```python
from build123d import *

# Parameters (mm, degrees)
SKETCH_1_R          = 30.5
EXTRUDE_1_DEPTH     = 12.6
SKETCH_2_R          = 32.75
EXTRUDE_2_DEPTH     = 22
SKETCH_3_R          = 29
EXTRUDE_3_DEPTH     = 5
EXTRUDE_START       = -1.1
EXTRUDE_4_DEPTH     = 10.6
SKETCH_5_R          = 1.5
CUT_EXTRUDE_1_DEPTH = 5
SKETCH_6_R          = 27.75
CUT_EXTRUDE_2_DEPTH = 2
CUT_EXTRUDE_START   = -1.2
CUT_EXTRUDE_3_DEPTH = 10.8


with BuildPart() as part:
    # 草图1 → 凸台-拉伸1 (new body)
    with BuildSketch(Plane.XY):
        Circle(SKETCH_1_R)
    extrude(amount=EXTRUDE_1_DEPTH)

    # 草图2 → 凸台-拉伸2 (add)
    with BuildSketch(Plane.XY.offset(12.6)):
        Circle(SKETCH_2_R)
    extrude(amount=EXTRUDE_2_DEPTH)

    # 草图3 → 凸台-拉伸3 (add)
    with BuildSketch(Plane.XY.offset(34.6)):
        Circle(SKETCH_3_R)
    extrude(amount=EXTRUDE_3_DEPTH)

    # 草图4 → 凸台-拉伸4 (add)
    with BuildSketch(Plane(origin=(0, 0, 0), x_dir=(-1, 0, 0), z_dir=(0, 0, -1)).offset(EXTRUDE_START)):
        with BuildLine():
            ThreePointArc((21.25, -21.878928219), (0, -30.5), (-21.25, -21.878928219))
            Line((-21.25, -21.878928219), (-21.25, -36.2))
            Line((-21.25, -36.2), (21.25, -36.2))
            Line((21.25, -36.2), (21.25, -21.878928219))
        make_face()
    extrude(amount=-EXTRUDE_4_DEPTH)

    # 草图5 → 切除-拉伸1 (cut)
    with BuildSketch(Plane.XZ.offset(36.2)):
        with Locations(Location((-18, 6.4, 0), (0, 0, 270))):
            Circle(SKETCH_5_R)
        with Locations(Location((18, 6.4, 0), (0, 0, 90))):
            Circle(SKETCH_5_R)
    extrude(amount=-CUT_EXTRUDE_1_DEPTH, mode=Mode.SUBTRACT)

    # 草图6 → 切除-拉伸2 (cut)
    with BuildSketch(Plane(origin=(0, 0, 0), x_dir=(-1, 0, 0), z_dir=(0, 0, -1))):
        Circle(SKETCH_6_R)
    extrude(amount=-CUT_EXTRUDE_2_DEPTH, mode=Mode.SUBTRACT)

    # 草图7 → 切除-拉伸3 (cut)
    with BuildSketch(Plane(origin=(0, 0, 0), x_dir=(-1, 0, 0), z_dir=(0, 0, -1)).offset(CUT_EXTRUDE_START)):
        with BuildLine():
            ThreePointArc((28.52384967, 10.8), (0, 30.5), (-28.52384967, 10.8))
            Line((-28.52384967, 10.8), (-27.988569095, 10.8))
            ThreePointArc((-27.988569095, 10.8), (0, 30), (27.988569095, 10.8))
            Line((27.988569095, 10.8), (28.52384967, 10.8))
        make_face()
    extrude(amount=-CUT_EXTRUDE_3_DEPTH, mode=Mode.SUBTRACT)


solid = part.part
```
The model under review builds one solid part; all positions refer to its coordinate system, in mm. A direction names the side the tool comes from. Give positions to 0.01 mm unless a question says otherwise; leave off trailing zeros. Write each loop counter-clockwise with the first axis right and the second up, starting at its lowest first coordinate (ties: lowest second). Pieces come first, ordered by that corner, then holes.
(1) Consider section D-D, the plane x = -18. Give the boundary of the cut face in (y, z), and give its area (3 significant figures).
(2) Tool access review of faces 1 (the cylindrical face through (-16.735, -33.735, 5.594)), 2 (the cylindrical face through (31.238, 9.837, 23.446)), 3 (the flat face through (21.25, -29, 6)), 4 (the cylindrical face through (0.505, 29.996, 6.524)), 5 (the flat face through (-21.25, -29, 6)): name each direction out of +Z, -Z, +X, -X, +Y, -Y from which nothing blocks a thin tool from reaching the whole face with its end or side.
(3) Consider section A-A, the plane y = 0. Give the boundary of the cut face in (x, z).
(4) For P1, Ø3, axis at x = 21, y = -22.5, coming from the +Z side; P2, Ø3, axis at y = -9.5, z = 15.5, coming from the +X side; P3, Ø1.5, axis at x = 18, z = 6.5, coming from the -Y side; P4, Ø3, axis at x = 24.5, y = 25, coming from the +Z side, all flat-tipped, find the tip position at first contact; note any pin that passes through.
(5) The part is to be moulded in two halves that separate along X. For faces 6 (the cylindrical face through (13.38, -25.73, 37.06)), 7 (the flat face through (0, 0, 2)), 8 (the flat face through (0.1, 30.2, 12)), say which applies: released by +X, released by -X, zero draft, split by the parting line, or undercut.
(6) To check wall thickness, follow L1, parallel to X at y = -32.6, z = 6.4; L2, parallel to Y at x = 0, z = 0.8; L3, parallel to Y at x = 0, z = 1.3. State the ranges of each line that lie inside material, in increasing order.
(7) Consider section B-B, the plane z = 6.4. Give the boundary of the cut face in (x, y).
(8) Consider section C-C, the plane x = -2. Give the boundary of the cut face in (y, z), and give its area (3 significant figures).
Returned:
1. outline: (-36.2, 1.1) - (-24.62, 1.1) - (-24.62, 0) - (-21.12, 0) - (-21.12, 2) - (21.12, 2) - (21.12, 0) - (24.62, 0) - (24.62, 1.2) - (24, 1.2) - (24, 12) - (24.62, 12) - (24.62, 12.6) - (27.36, 12.6) - (27.36, 34.6) - (22.74, 34.6) - (22.74, 39.6) - (-22.74, 39.6) - (-22.74, 34.6) - (-27.36, 34.6) - (-27.36, 12.6) - (-24.62, 12.6) - (-24.62, 11.7) - (-36.2, 11.7) - (-36.2, 7.9) - (-31.2, 7.9) - (-31.2, 4.9) - (-36.2, 4.9) - close
1. area: 2,070 mm2
2. face 1: -Y
2. face 2: +Z
2. face 3: -Z, +X, -Y
2. face 4: +Y
2. face 5: -Z, -X, -Y
3. outline: (-32.75, 12.6) - (-30.5, 12.6) - (-30.5, 0) - (-27.75, 0) - (-27.75, 2) - (27.75, 2) - (27.75, 0) - (30.5, 0) - (30.5, 12.6) - (32.75, 12.6) - (32.75, 34.6) - (29, 34.6) - (29, 39.6) - (-29, 39.6) - (-29, 34.6) - (-32.75, 34.6) - close
4. P1: stops at z = 34.6
4. P2: stops at x = 31.76
4. P3: stops at y = -31.2
4. P4: passes through
5. face 6: split by the parting line
5. face 7: undercut
5. face 8: zero draft
6. L1: x = -21.25 to -19.5, -16.5 to 16.5, 19.5 to 21.25
6. L2: y = -30.5 to -27.75, 27.75 to 30.5
6. L3: y = -36.2 to -27.75, 27.75 to 30
7. outline: (-28.52, 10.8) arc R30.5 ccw to (-21.25, -21.88) - (-21.25, -36.2) - (-19.5, -36.2) - (-19.5, -31.2) - (-16.5, -31.2) - (-16.5, -36.2) - (16.5, -36.2) - (16.5, -31.2) - (19.5, -31.2) - (19.5, -36.2) - (21.25, -36.2) - (21.25, -21.88) arc R30.5 ccw to (28.52, 10.8) - (27.99, 10.8) arc R30 ccw to (-27.99, 10.8) - close
8. outline: (-36.2, 1.1) - (-30.43, 1.1) - (-30.43, 0) - (-27.68, 0) - (-27.68, 2) - (27.68, 2) - (27.68, 0) - (30.43, 0) - (30.43, 1.2) - (29.93, 1.2) - (29.93, 12) - (30.43, 12) - (30.43, 12.6) - (32.69, 12.6) - (32.69, 34.6) - (28.93, 34.6) - (28.93, 39.6) - (-28.93, 39.6) - (-28.93, 34.6) - (-32.69, 34.6) - (-32.69, 12.6) - (-30.43, 12.6) - (-30.43, 11.7) - (-36.2, 11.7) - close
8. area: 2,440 mm2
